Autodesk Inventor part; units mm, degrees
ref_plane "YZ Plane" through (0, 0, 0) normal (1, 0, 0) x (0, 1, 0)
ref_plane "XZ Plane" through (0, 0, 0) normal (0, 1, 0) x (-1, 0, 0)
ref_plane "XY Plane" through (0, 0, 0) normal (0, 0, 1) x (1, 0, 0)
sketch "Sketch1" plane through (0, 0, 0) normal (0, 0, 1) x (1, 0, 0)
  circle A0 centre (0, 0) radius 57.5
  circle A1 centre (0, 0) radius 60.5
  line L0 (-40.5, 60.5) -> (40.5, 60.5)
  line L1 (60.5, 40.5) -> (60.5, -40.5)
  line L2 (40.5, -60.5) -> (-40.5, -60.5)
  line L3 (-60.5, -40.5) -> (-60.5, 40.5)
  arc A2 (-40.5, 60.5) -> (-60.5, 40.5) centre (-40.5, 40.5) ccw
  arc A3 (60.5, 40.5) -> (40.5, 60.5) centre (40.5, 40.5) ccw
  arc A4 (40.5, -60.5) -> (60.5, -40.5) centre (40.5, -40.5) ccw
  arc A5 (-60.5, -40.5) -> (-40.5, -60.5) centre (-40.5, -40.5) ccw
  dimension "d0" = 115
  dimension "d1" = 121
  dimension "d2" = 20
extrude "Extrusion1" add sketch "Sketch1" along normal blind 7.7
sketch "Sketch3" plane through (0, 0, 7.7) normal (0, 0, 1) x (1, 0, 0)
  circle A0 centre (-48.4934, -48.5066) radius 2.65
  circle A1 centre (-37.2752, -53.25) radius 2.15
  circle A2 centre (-53.2398, -37.2897) radius 2.15
  circle A3 centre (-53.25, 37.2752) radius 2.15
  circle A4 centre (-48.5066, 48.4934) radius 2.65
  circle A5 centre (-37.2897, 53.2398) radius 2.15
  circle A6 centre (53.2398, 37.2897) radius 2.15
  circle A7 centre (48.4934, 48.5066) radius 2.65
  circle A8 centre (37.2752, 53.25) radius 2.15
  circle A9 centre (53.25, -37.2752) radius 2.15
  circle A10 centre (48.5066, -48.4934) radius 2.65
  circle A11 centre (37.2897, -53.2398) radius 2.15
  point P0 (0, 0)
extrude "Extrusion3" cut sketch "Sketch3" against normal through all
sketch "Sketch4" plane through (0, 0, 7.7) normal (0, 0, 1) x (1, 0, 0)
  circle A0 centre (0, 0) radius 29
  line L0 (9.6493, -46.097) -> (11.4281, -54.5943)
  arc A1 (-7.99, -55.2023) -> (11.4281, -54.5943) centre (0, 0) ccw
  line L1 (-7.99, -55.2023) -> (-6.7464, -46.6104)
  arc A2 (-6.7464, -46.6104) -> (9.6493, -46.097) centre (0, 0) ccw
  line L2 (-26.2539, 39.0996) -> (-31.0934, 46.307)
  arc A3 (-8.5912, 55.112) -> (-31.0934, 46.307) centre (0, 0) ccw
  line L3 (-8.5912, 55.112) -> (-7.254, 46.5341)
  arc A4 (-7.254, 46.5341) -> (-26.2539, 39.0996) centre (0, 0) ccw
  line L4 (53.6989, -15.0854) -> (45.341, -12.7375)
  arc A5 (45.341, -12.7375) -> (47.0109, 2.8322) centre (0, 0) ccw
  line L5 (47.0109, 2.8322) -> (55.6766, 3.3542)
  arc A6 (53.6989, -15.0854) -> (55.6766, 3.3542) centre (0, 0) ccw
  line L6 (54.7773, 10.5158) -> (46.2516, 8.8791)
  arc A7 (46.2516, 8.8791) -> (35.4257, 31.0334) centre (0, 0) ccw
  line L7 (35.4257, 31.0334) -> (41.9558, 36.7539)
  arc A8 (54.7773, 10.5158) -> (41.9558, 36.7539) centre (0, 0) ccw
  line L8 (-15.7851, -44.372) -> (-18.6949, -52.5513)
  arc A9 (-35.715, -42.8436) -> (-18.6949, -52.5513) centre (0, 0) ccw
  line L9 (-35.715, -42.8436) -> (-30.1562, -36.1753)
  arc A10 (-30.1562, -36.1753) -> (-15.7851, -44.372) centre (0, 0) ccw
  line L10 (11.2228, 54.6369) -> (9.4761, 46.133)
  arc A11 (9.4761, 46.133) -> (-4.3919, 46.8909) centre (0, 0) ccw
  line L11 (-4.3919, 46.8909) -> (-5.2015, 55.5345)
  arc A12 (11.2228, 54.6369) -> (-5.2015, 55.5345) centre (0, 0) ccw
  line L12 (38.5468, -40.3148) -> (32.5472, -34.04)
  arc A13 (32.5472, -34.04) -> (42.2602, -20.7876) centre (0, 0) ccw
  line L13 (42.2602, -20.7876) -> (50.0502, -24.6195)
  arc A14 (38.5468, -40.3148) -> (50.0502, -24.6195) centre (0, 0) ccw
  line L14 (36.8913, 41.835) -> (31.1494, 35.3237)
  arc A15 (31.1494, 35.3237) -> (19.437, 42.8982) centre (0, 0) ccw
  line L15 (19.437, 42.8982) -> (23.0199, 50.8058)
  arc A16 (36.8913, 41.835) -> (23.0199, 50.8058) centre (0, 0) ccw
  line L16 (-34.6849, -31.8592) -> (-41.0785, -37.7319)
  arc A17 (-54.5943, -11.4281) -> (-41.0785, -37.7319) centre (0, 0) ccw
  line L17 (-54.5943, -11.4281) -> (-46.097, -9.6493)
  arc A18 (-46.097, -9.6493) -> (-34.6849, -31.8592) centre (0, 0) ccw
  circle A19 centre (37.2752, 53.25) radius 2.15
  circle A20 centre (16.4961, 28.5811) radius 1.25
  circle A21 centre (-37.2752, -53.25) radius 2.15
  circle A22 centre (-37.2897, 53.2398) radius 2.15
  circle A23 centre (48.5066, -48.4934) radius 2.65
  circle A24 centre (-48.4934, -48.5066) radius 2.65
  circle A25 centre (-53.25, 37.2752) radius 2.15
  circle A26 centre (-53.2398, -37.2897) radius 2.15
  circle A27 centre (16.5039, -28.5766) radius 1.25
  circle A28 centre (53.2398, 37.2897) radius 2.15
  circle A29 centre (53.25, -37.2752) radius 2.15
  circle A30 centre (-16.4961, -28.5811) radius 1.25
  circle A31 centre (-16.5039, 28.5766) radius 1.25
  circle A32 centre (48.4934, 48.5066) radius 2.65
  circle A33 centre (-48.5066, 48.4934) radius 2.65
  circle A34 centre (-33, -0.0045) radius 1.25
  circle A35 centre (37.2897, -53.2398) radius 2.15
  circle A36 centre (33, 0.0045) radius 1.25
  line L18 (-59.5162, 33.2815) -> (-60.5047, 34.4337)
  line L19 (-59.5162, 33.2815) -> (-50.1662, 31.842)
  line L20 (-43.8555, 34.4649) -> (-50.1662, 31.842)
  arc A37 (-39.7545, 39.1244) -> (-43.8555, 34.4649) centre (0, 0) ccw
  line L21 (-39.7545, 39.1244) -> (-33.5669, 33.0349)
  arc A38 (-33.5669, 33.0349) -> (-47.0756, -1.3908) centre (0, 0) ccw
  line L22 (-47.0756, -1.3908) -> (-55.7533, -1.6472)
  line L23 (-55.7533, -1.6472) -> (-59.4998, -1.6477)
  line L24 (-60.4996, -2.6478) -> (-59.4998, -1.6477)
  line L25 (-60.4996, -2.6478) -> (-60.4945, -40.5083)
  arc A39 (-60.4945, -40.5083) -> (-40.4917, -60.5055) centre (-40.4945, -40.5055) ccw
  line L26 (-40.4917, -60.5055) -> (40.5083, -60.4945)
  arc A40 (40.5083, -60.4945) -> (60.5055, -40.4917) centre (40.5055, -40.4945) ccw
  line L27 (60.5055, -40.4917) -> (60.4945, 40.5083)
  arc A41 (60.4945, 40.5083) -> (40.4917, 60.5055) centre (40.4945, 40.5055) ccw
  line L28 (40.4917, 60.5055) -> (-40.5083, 60.4945)
  arc A42 (-40.5083, 60.4945) -> (-60.5055, 40.4917) centre (-40.5055, 40.4945) ccw
  line L29 (-60.5055, 40.4917) -> (-60.5047, 34.4337)
  circle A43 centre (-53.2398, -37.2897) radius 2.15
  circle A44 centre (53.2398, 37.2897) radius 2.15
  circle A45 centre (48.5066, -48.4934) radius 2.65
  circle A46 centre (37.2897, -53.2398) radius 2.15
  circle A47 centre (-37.2897, 53.2398) radius 2.15
  circle A48 centre (-48.4934, -48.5066) radius 2.65
  circle A49 centre (-53.25, 37.2752) radius 2.15
  circle A50 centre (48.4934, 48.5066) radius 2.65
  circle A51 centre (53.25, -37.2752) radius 2.15
  circle A52 centre (37.2752, 53.25) radius 2.15
  circle A53 centre (-48.5066, 48.4934) radius 2.65
  circle A54 centre (-37.2752, -53.25) radius 2.15
  line L30 (-60.5, 40.5) -> (-60.5, -40.5)
  arc A55 (-60.5, -40.5) -> (-40.5, -60.5) centre (-40.5, -40.5) ccw
  line L31 (-40.5, -60.5) -> (40.5, -60.5)
  arc A56 (40.5, -60.5) -> (60.5, -40.5) centre (40.5, -40.5) ccw
  line L32 (60.5, -40.5) -> (60.5, 40.5)
  arc A57 (60.5, 40.5) -> (40.5, 60.5) centre (40.5, 40.5) ccw
  line L33 (40.5, 60.5) -> (-40.5, 60.5)
  arc A58 (-40.5, 60.5) -> (-60.5, 40.5) centre (-40.5, 40.5) ccw
  circle A59 centre (0, 0) radius 57.5
  point P0 (-54.6384, -54.6459)
  point P1 (0.0041, -60.5)
  point P2 (54.6459, -54.6384)
  point P3 (60.5, 0.0041)
  point P4 (54.6384, 54.6459)
  point P5 (-0.0041, 60.5)
  point P6 (-54.6459, 54.6384)
  point P7 (-60.5, 34.4282)
  point P8 (-57.4764, -1.6474)
  point P9 (-46.9668, 33.1718)
extrude "Extrusion4" add sketch "Sketch4" along normal blind 0.7 contours L19 L20 A59 L23 L24 L30 L18 | L18 L30 A58 A42 L28 L33 A57 A41 L27 L32 A56 A40 L26 L31 A55 A39 L25 L24 L23 A59 L20 L19 | L25 A39 A55 L30 | A59 L23 L22 A38 L21 A37 L20 | A58 L33 L28 A42 | L26 A40 A56 L31 | A57 L32 L27 A41 picked at (17.5819, -42.3508)
sketch "Sketch5" plane through (0, 0, 8.4) normal (0, 0, 1) x (1, 0, 0)
  circle A0 centre (-33, -0.0045) radius 1.25
  circle A1 centre (-33, -0.0045) radius 1.75
  circle A2 centre (-16.4961, -28.5811) radius 1.75
  circle A3 centre (16.5039, -28.5766) radius 1.75
  circle A4 centre (33, 0.0045) radius 1.75
  circle A5 centre (16.4961, 28.5811) radius 1.75
  circle A6 centre (-16.5039, 28.5766) radius 1.75
  point P0 (0, 0)
  dimension "d30" = 3.5
  dimension "d33" = 360
extrude "Extrusion5" cut sketch "Sketch5" against normal through all contours A0 | A1 | A2 | A3 | A4 | A5 | A6
sketch "Sketch6" plane through (0, 0, 7.7) normal (0, 0, -1) x (-1, 0, 0)
  circle A0 centre (0, 0) radius 35
  circle A1 centre (-33, 0.0045) radius 1.75
  circle A2 centre (33, -0.0045) radius 1.75
  circle A3 centre (-16.5039, -28.5766) radius 1.75
  circle A4 centre (-16.4961, 28.5811) radius 1.75
  circle A5 centre (16.5039, 28.5766) radius 1.75
  circle A6 centre (16.4961, -28.5811) radius 1.75
  circle A7 centre (0, 0) radius 29
  line L0 (7.99, -55.2023) -> (6.7464, -46.6104)
  arc A8 (-11.4281, -54.5943) -> (7.99, -55.2023) centre (0, 0) ccw
  line L1 (-9.6493, -46.097) -> (-11.4281, -54.5943)
  arc A9 (-9.6493, -46.097) -> (6.7464, -46.6104) centre (0, 0) ccw
  line L2 (8.5912, 55.112) -> (7.254, 46.5341)
  arc A10 (31.0934, 46.307) -> (8.5912, 55.112) centre (0, 0) ccw
  line L3 (26.2539, 39.0996) -> (31.0934, 46.307)
  arc A11 (26.2539, 39.0996) -> (7.254, 46.5341) centre (0, 0) ccw
  line L4 (-53.6989, -15.0854) -> (-45.341, -12.7375)
  arc A12 (-55.6766, 3.3542) -> (-53.6989, -15.0854) centre (0, 0) ccw
  line L5 (-47.0109, 2.8322) -> (-55.6766, 3.3542)
  arc A13 (-47.0109, 2.8322) -> (-45.341, -12.7375) centre (0, 0) ccw
  line L6 (-54.7773, 10.5158) -> (-46.2516, 8.8791)
  arc A14 (-41.9558, 36.7539) -> (-54.7773, 10.5158) centre (0, 0) ccw
  line L7 (-35.4257, 31.0334) -> (-41.9558, 36.7539)
  arc A15 (-35.4257, 31.0334) -> (-46.2516, 8.8791) centre (0, 0) ccw
  line L8 (35.715, -42.8436) -> (30.1562, -36.1753)
  arc A16 (18.6949, -52.5513) -> (35.715, -42.8436) centre (0, 0) ccw
  line L9 (15.7851, -44.372) -> (18.6949, -52.5513)
  arc A17 (15.7851, -44.372) -> (30.1562, -36.1753) centre (0, 0) ccw
  line L10 (-11.2228, 54.6369) -> (-9.4761, 46.133)
  arc A18 (5.2015, 55.5345) -> (-11.2228, 54.6369) centre (0, 0) ccw
  line L11 (4.3919, 46.8909) -> (5.2015, 55.5345)
  arc A19 (4.3919, 46.8909) -> (-9.4761, 46.133) centre (0, 0) ccw
  line L12 (-38.5468, -40.3148) -> (-32.5472, -34.04)
  arc A20 (-50.0502, -24.6195) -> (-38.5468, -40.3148) centre (0, 0) ccw
  line L13 (-42.2602, -20.7876) -> (-50.0502, -24.6195)
  arc A21 (-42.2602, -20.7876) -> (-32.5472, -34.04) centre (0, 0) ccw
  line L14 (-36.8913, 41.835) -> (-31.1494, 35.3237)
  arc A22 (-23.0199, 50.8058) -> (-36.8913, 41.835) centre (0, 0) ccw
  line L15 (-19.437, 42.8982) -> (-23.0199, 50.8058)
  arc A23 (-19.437, 42.8982) -> (-31.1494, 35.3237) centre (0, 0) ccw
  line L16 (54.5943, -11.4281) -> (46.097, -9.6493)
  arc A24 (41.0785, -37.7319) -> (54.5943, -11.4281) centre (0, 0) ccw
  line L17 (34.6849, -31.8592) -> (41.0785, -37.7319)
  arc A25 (34.6849, -31.8592) -> (46.097, -9.6493) centre (0, 0) ccw
  arc A26 (46.9668, 33.1718) -> (57.4764, -1.6474) centre (0, 0) ccw
  line L18 (55.7533, -1.6472) -> (57.4764, -1.6474)
  line L19 (47.0756, -1.3908) -> (55.7533, -1.6472)
  arc A27 (47.0756, -1.3908) -> (33.5669, 33.0349) centre (0, 0) ccw
  line L20 (39.7545, 39.1244) -> (33.5669, 33.0349)
  arc A28 (43.8555, 34.4649) -> (39.7545, 39.1244) centre (0, 0) ccw
  line L21 (46.9668, 33.1718) -> (43.8555, 34.4649)
  dimension "d37" = 70
extrude "Extrusion6" add sketch "Sketch6" along normal blind 0.5 contours A0
sketch "Sketch8" plane through (0, 0, 8.4) normal (0, 0, 1) x (1, 0, 0)
  circle A0 centre (0, 0) radius 44
  dimension "d46" = 88
extrude "Extrusion8" cut sketch "Sketch8" against normal through all
sketch "Sketch9" plane through (-40.5, 60.5, 0) normal (0, 1, 0) x (1, 0, 0)
  circle A0 centre (10.5, -4.15) radius 2.15
  line L0 (101, 0) -> (101, -8.4)
  line L1 (-20, 0) -> (-20, -8.4)
  line L2 (81, -8.4) -> (0, -8.4)
  circle A1 centre (70.5, -4.15) radius 2.15
  point P0 (40.5, 0)
  dimension "d49" = 4.3
  dimension "d50" = 121
  dimension "d51" = 4.25
  dimension "d52" = 30.5
  dimension "d55" = 60
extrude "Extrusion9" cut sketch "Sketch9" against normal blind 10
sketch "Sketch10" plane through (-40.5, -60.5, 0) normal (0, -1, 0) x (1, 0, 0)
  circle A0 centre (10.5, 4.15) radius 2.15
  circle A1 centre (70.5, 4.15) radius 2.15
  point P0 (40.5, 0)
extrude "Extrusion10" cut sketch "Sketch10" against normal blind 10
sketch "Sketch11" plane through (60.5, -40.5, 0) normal (1, 0, 0) x (0, 0, -1)
  circle A0 centre (-4.15, 10.5) radius 2.15
  line L0 (0, 101) -> (-8.4, 101)
  line L1 (0, -20) -> (-8.4, -20)
  line L2 (-8.4, 0) -> (-8.4, -20)
  circle A1 centre (-4.15, 70.5) radius 2.15
  point P0 (0, 40.5)
  dimension "d64" = 4.3
  dimension "d65" = 121
  dimension "d66" = 4.25
  dimension "d67" = 30.5
  dimension "d70" = 60
extrude "Extrusion11" cut sketch "Sketch11" against normal blind 10
sketch "Sketch12" plane through (-60.5, -40.5, 0) normal (-1, 0, 0) x (0, 0, 1)
  circle A0 centre (4.15, 70.5) radius 2.15
  circle A1 centre (4.15, 10.5) radius 2.15
  point P0 (0, 40.5)
extrude "Extrusion12" cut sketch "Sketch12" against normal blind 10
properties part number "stator_center_01_p" material "PC/ABS Plastic"
Read the model definition and answer for the solid it produces. Units are mm, in the model's axes. A direction names the side the tool comes from. Coordinates: 2 decimals unless noted, no trailing zeros. Order: outer loops, then holes, each group sorted by start corner. A loop starts at its lowest first (then second) coordinate and runs counter-clockwise, first axis right, second up. Notation, with made-up numbers: (10.5, 44.5) - (19.5, 44.5) arc R28 ccw to (19.5, 70.5) - close; hole circle Ø7 at (5, 50). An arc over 180 degrees is marked (long way). Answer as a JSON object with one key per item and string values. Group by question number.
Item 1: Section B-B (x = 0) is taken. Give the vertices of the cut face in (y, z), plus the area to 3 significant figures.
Item 2: Section D-D (x = -24) is taken. Give the vertices of the cut face in (y, z), plus the area to 3 significant figures.
Item 3: Consider probe 1 along Y at (x, z) = (-36, 7); probe 2 along Y at (x, z) = (-35.5, 6.5); probe 3 along Y at (x, z) = (32.5, 3.25). Determine where each line is inside the solid, lowest interval first. Write a range as from..to.
Item 4: Flat-ended cylindrical pins translate along their axes: P1, Ø4, axis at x = 48.51, y = -48.49, coming from the +Z side; P2, Ø1.3, axis at y = -29, z = 4.5, coming from the -X side; P3, Ø7, axis at x = -53.25, y = 37.28, coming from the -Z side; P4, Ø1.5, axis at x = -44.5, z = 2, coming from the +Y side. Find the tip coordinate at first contact, or state that the pin passes through.
Item 5: The mould has two halves that part along Z. Classify faces 4 (the face through (0, 59, 0)), 5 (the face through (-27.95, 55.57, 3.5)), 6 (the face through (35.59, -37.22, 8.05)): +Z half, -Z half, draft (parallel to the pull), parting line (faces both ways), or undercut.
Item 6: A tool of negligible diameter and unlimited length cuts with its end or side. For faces 1 (the face through (-30, 50.5, 4)), 2 (the face through (-27.95, -55.57, 4.8)), 3 (the face through (38.645, 33.854, 8.045)), from which of +Z, -Z, +X, -X, +Y, -Y can it reach the whole face along a straight path? Write none if from no direction.
Item 7: Section C-C (y = -30) is taken. Give the vertices of the cut face in (x, z).
Item 8: Section A-A (x = 17) is taken. Give the vertices of the cut face in (y, z), plus the area to 3 significant figures.
Results are:
{
 "1": {"outline": "(-60.5, 0) - (-57.5, 0) - (-57.5, 7.7) - (-55.78, 7.7) - (-55.78, 8.4) - (-60.5, 8.4) - close; (-47.1, 7.7) - (-44, 7.7) - (-44, 8.4) - (-47.1, 8.4) - close; (44, 7.7) - (47.1, 7.7) - (47.1, 8.4) - (44, 8.4) - close; (55.78, 7.7) - (57.5, 7.7) - (57.5, 0) - (60.5, 0) - (60.5, 8.4) - (55.78, 8.4) - close", "area": "57.1 mm^2"},
 "2": {"outline": "(-60.5, 0) - (-52.25, 0) - (-52.25, 7.7) - (-50.35, 7.7) - (-50.35, 8.4) - (-60.5, 8.4) - close; (-40.52, 7.7) - (-36.88, 7.7) - (-36.88, 8.4) - (-40.52, 8.4) - close; (36.88, 7.7) - (40.52, 7.7) - (40.52, 8.4) - (36.88, 8.4) - close; (50.35, 7.7) - (52.25, 7.7) - (52.25, 0) - (60.5, 0) - (60.5, 8.4) - (50.35, 8.4) - close", "area": "146 mm^2"},
 "3": {"probe 1": "y = -60.5..-54.98, -51.52..-44.84, 44.84..51.52, 54.96..60.5", "probe 2": "y = -60.5..-54.46, -52.04..-45.23, 45.23..52.05, 54.43..60.5", "probe 3": "y = -60.5..-47.43, 47.43..60.5"},
 "4": {"P1": "passes through", "P2": "stops at x = -50.5", "P3": "stops at z = 0", "P4": "stops at y = 60.23"},
 "5": {"face 4": "-Z half", "face 5": "undercut", "face 6": "draft"},
 "6": {"face 1": "+Y", "face 2": "-Y", "face 3": "+Z, -Z"},
 "7": {"outline": "(-60.5, 0) - (-49.05, 0) - (-49.05, 7.7) - (-47.02, 7.7) - (-47.02, 8.4) - (-60.5, 8.4) - (-60.5, 6.3) - (-50.5, 6.3) - (-50.5, 2) - (-60.5, 2) - close; (-36.3, 7.7) - (-32.19, 7.7) - (-32.19, 8.4) - (-36.3, 8.4) - close; (32.19, 7.7) - (36.3, 7.7) - (36.3, 8.4) - (32.19, 8.4) - close; (47.02, 7.7) - (49.05, 7.7) - (49.05, 0) - (60.5, 0) - (60.5, 2) - (50.5, 2) - (50.5, 6.3) - (60.5, 6.3) - (60.5, 8.4) - (47.02, 8.4) - close"},
 "8": {"outline": "(-60.5, 0) - (-54.93, 0) - (-54.93, 7.7) - (-40.58, 7.7) - (-40.58, 8.4) - (-60.5, 8.4) - close; (40.58, 7.7) - (54.93, 7.7) - (54.93, 0) - (60.5, 0) - (60.5, 8.4) - (40.58, 8.4) - close", "area": "114 mm^2"}
}
